```python
from build123d import *

# Parameters (mm, degrees)
F1_DEPTH = 76.2
F2_DEPTH = 12.7
F4_DEPTH = 1270
F6_DEPTH = 70.612
F7_START = -12.7
F7_DEPTH = 43.434


with BuildPart() as f1:
    # F0 (on Front) → F1 (new body, symmetric)
    with BuildSketch(Plane.XZ):
        Polygon((0, 203.2), (0, 0), (254, 0), (254, 25.4), (63.5, 25.4), (25.4, 25.4), (25.4, 76.2), (25.4, 203.2), align=None)
    extrude(amount=F1_DEPTH, both=True)

    # F0 (on Front) → F2 (join, symmetric)
    with BuildSketch(Plane.XZ):
        Polygon((63.5, 25.4), (25.4, 76.2), (25.4, 25.4), align=None)
    extrude(amount=F2_DEPTH, both=True)

    # F3 (on face) → F4 (cut, symmetric)
    with BuildSketch(Plane(origin=(0, 0, 0), x_dir=(0, -1, 0), z_dir=(-1, 0, 0))):
        with BuildLine():
            Line((-76.2, 203.2), (-76.2, 127))
            ThreePointArc((-76.2, 127), (-53.8815367264, 180.8815367264), (0, 203.2))
            Line((0, 203.2), (-76.2, 203.2))
        make_face()
        with BuildLine():
            Line((76.2, 203.2), (0, 203.2))
            ThreePointArc((0, 203.2), (53.8815367264, 180.8815367264), (76.2, 127))
            Line((76.2, 127), (76.2, 203.2))
        make_face()
        with BuildLine():
            ThreePointArc((38.1, 127), (-26.9407683632, 153.9407683632), (0, 88.9))
            ThreePointArc((0, 88.9), (26.9407683632, 100.0592316368), (38.1, 127))
        make_face()
    extrude(amount=F4_DEPTH, both=True, mode=Mode.SUBTRACT)

    # F5 (on face) → F6 (cut)
    with BuildSketch(Plane(origin=(0, 0, 0), x_dir=(1, 0, 0), z_dir=(0, 0, -1))):
        with BuildLine():
            ThreePointArc((203.2, 76.2), (212.1802561211, 72.4802561211), (215.9, 63.5))
            Line((215.9, 63.5), (215.9, 38.1))
            ThreePointArc((215.9, 38.1), (219.6197438789, 29.1197438789), (228.6, 25.4))
            Line((228.6, 25.4), (241.3, 25.4))
            Line((241.3, 25.4), (254, 25.4))
            Line((254, 25.4), (254, 76.2))
            Line((254, 76.2), (203.2, 76.2))
        make_face()
        with BuildLine():
            ThreePointArc((88.9, 38.1), (92.6197438789, 29.1197438789), (101.6, 25.4))
            Line((101.6, 25.4), (177.8, 25.4))
            ThreePointArc((177.8, 25.4), (186.7802561211, 29.1197438789), (190.5, 38.1))
            ThreePointArc((190.5, 38.1), (186.7802561211, 47.0802561211), (177.8, 50.8))
            Line((177.8, 50.8), (101.6, 50.8))
            ThreePointArc((101.6, 50.8), (92.6197438789, 47.0802561211), (88.9, 38.1))
        make_face()
        with BuildLine():
            ThreePointArc((101.6, -25.4), (92.6197438789, -29.1197438789), (88.9, -38.1))
            ThreePointArc((88.9, -38.1), (92.6197438789, -47.0802561211), (101.6, -50.8))
            Line((101.6, -50.8), (177.8, -50.8))
            ThreePointArc((177.8, -50.8), (186.7802561211, -47.0802561211), (190.5, -38.1))
            ThreePointArc((190.5, -38.1), (186.7802561211, -29.1197438789), (177.8, -25.4))
            Line((177.8, -25.4), (101.6, -25.4))
        make_face()
        with BuildLine():
            Line((254, -25.4), (241.3, -25.4))
            Line((241.3, -25.4), (228.6, -25.4))
            ThreePointArc((228.6, -25.4), (219.6197438789, -29.1197438789), (215.9, -38.1))
            Line((215.9, -38.1), (215.9, -63.5))
            ThreePointArc((215.9, -63.5), (212.1802561211, -72.4802561211), (203.2, -76.2))
            Line((203.2, -76.2), (254, -76.2))
            Line((254, -76.2), (254, -25.4))
        make_face()
    extrude(amount=-F6_DEPTH, mode=Mode.SUBTRACT)

    # F5 (on face) → F7 (cut)
    with BuildSketch(Plane(origin=(0, 0, 0), x_dir=(1, 0, 0), z_dir=(0, 0, -1)).offset(F7_START)):
        with BuildLine():
            Line((254, 0), (254, 12.7))
            Line((254, 12.7), (228.6, 12.7))
            ThreePointArc((228.6, 12.7), (219.6197438789, 8.9802561211), (215.9, 0))
            ThreePointArc((215.9, 0), (219.6197438789, -8.9802561211), (228.6, -12.7))
            Line((228.6, -12.7), (254, -12.7))
            Line((254, -12.7), (254, 0))
        make_face()
    extrude(amount=-F7_DEPTH, mode=Mode.SUBTRACT)


solid = f1.part
```
Geometry check sheet. Reference: the model listing, model coordinates, mm. A direction names the side the tool comes from. Coordinates: 2 decimals unless noted, no trailing zeros. Write each loop counter-clockwise with the first axis right and the second up, starting at its lowest first coordinate (ties: lowest second). Pieces come first, ordered by that corner, then holes. Notation, with made-up numbers: (8.25, -37.5) -> (34.25, -37.5) arc R22 ccw to (34.25, -1.5) -> close; hole circle Ø11 at (39.25, 8.25). An arc over 180 degrees is marked (long way). Use CSV: the item, a comma, the result in double quotes. Start each with the question number.
Item 1: Depth check by flat-ended pin: pin 1 Ø7.5 at (x, z) = (243.5, 11.5) entering from -Y; pin 2 Ø3 at (x, y) = (129.5, -59.5) entering from -Z; pin 3 Ø7.5 at (x, y) = (242, -4.5) entering from +Z; pin 4 Ø20.5 at (y, z) = (-45.5, 16) entering from +X. Enter the tip coordinate at first touch or a pass-through.
Item 2: Cross-section at B-B, the plane y = -7. Record the cut outline in (x, z).
Item 3: Thickness scan on line 1 (Y direction, x = 15, z = 127); line 2 (X direction, y = -43.5, z = 72.5); line 3 (Y direction, x = 24, z = 193). Record the ranges inside material, lowest first.
Item 4: Cross-section at C-C, the plane x = 58. Record the cut outline in (y, z), plus the area to 3 significant figures.
Item 5: Cross-section at D-D, the plane x = 19. Record the cut outline in (y, z).
Item 6: Mould release check, pull along Z, two halves, no side actions. Record for faces 6 (the flat face through (140, 25.4, 13)), 7 (the cylindrical face through (12.522, -1.675, 165.063)), 8 (the flat face through (44.72, -0.18, 50.44)): released by +Z, released by -Z, zero draft, split by the parting line, or undercut.
Item 7: Cross-section at A-A, the plane z = 152. Record the cut outline in (x, y), plus the area to 3 significant figures.
Item 8: Set-up check for faces 1 (the flat face through (215.9, -51, 13)), 2 (the flat face through (215.9, 51, 13)), 3 (the flat face through (241, 12.7, 19)), 4 (the flat face through (0, -1, 80)), 5 (the flat face through (140, -50.8, 13)): record each of +Z, -Z, +X, -X, +Y, -Y from which the full face is reachable in a straight line by a thin tool's end or side.
Answers:
1,pin 1,"y = -25.4"
1,pin 2,"z = 0"
1,pin 3,"z = 12.7"
1,pin 4,"x = 216.22"
2,outline,"(0, 0) -> (254, 0) -> (254, 12.7) -> (218, 12.7) -> (218, 25.4) -> (63.5, 25.4) -> (25.4, 76.2) -> (25.4, 89.55) -> (0, 89.55) -> close; (0, 164.45) -> (25.4, 164.45) -> (25.4, 202.88) -> (0, 202.88) -> close"
3,line 1,"-76.2 to -38.1, 38.1 to 76.2"
3,line 2,"0 to 25.4"
3,line 3,"-38.08 to 38.08"
4,outline,"(-76.2, 0) -> (76.2, 0) -> (76.2, 25.4) -> (12.7, 25.4) -> (12.7, 32.73) -> (-12.7, 32.73) -> (-12.7, 25.4) -> (-76.2, 25.4) -> close"
4,area,"4,060 mm^2"
5,outline,"(-76.2, 0) -> (76.2, 0) -> (76.2, 127) arc R76.2 ccw to (-76.2, 127) -> close; hole circle Ø76.2 at (0, 127)"
6,face 6,"zero draft"
6,face 7,"undercut"
6,face 8,"released by +Z"
7,outline,"(0, -71.98) -> (25.4, -71.98) -> (25.4, -28.75) -> (0, -28.75) -> close; (0, 28.75) -> (25.4, 28.75) -> (25.4, 71.98) -> (0, 71.98) -> close"
7,area,"2,200 mm^2"
8,face 1,"+Z, -Z, +X, -Y"
8,face 2,"+Z, -Z, +X, +Y"
8,face 3,"+Z, +X"
8,face 4,"+Z, -Z, -X, +Y, -Y"
8,face 5,"+Z, -Z"
